```python
from build123d import *

# Parameters (mm, degrees)
SKETCH1_R           = 102.9
BOSS_EXTRUDE1_DEPTH = 230
BOSS_EXTRUDE1_DRAFT = -3
SHELL2_T            = -1


with BuildPart() as part:
    # Sketch1 → Boss-Extrude1 (with draft: the straight prism first)
    with BuildSketch(Plane(origin=(0, 0, 0), x_dir=(1, 0, 0), z_dir=(0, 1, 0))):
        Circle(SKETCH1_R)
    extrude(amount=BOSS_EXTRUDE1_DEPTH)
    # Boss-Extrude1: the draft: its side faces are tilted about the plane it starts from
    boss_extrude1_sides = [part.faces().sort_by_distance(p)[0] for p in [
        (-102.9, 115, 0),
    ]]
    draft(boss_extrude1_sides, Plane(origin=(0, 0, 0), x_dir=(1, 0, 0), z_dir=(0, 1, 0)), BOSS_EXTRUDE1_DRAFT)

    # Shell2
    shell2_openings = [part.faces().sort_by_distance(p)[0] for p in [
        (0, 230, 0),
    ]]
    offset(amount=SHELL2_T, openings=shell2_openings, kind=Kind.INTERSECTION)

    # Sketch4 → Revolve2 (revolve)
    with BuildSketch(Plane.XY, mode=Mode.PRIVATE) as revolve2_sk:
        Polygon((114.953789235, 230), (125.477867028, 230), (124.953789235, 220), (122.849117323, 220), (123.268523203, 228.00274093), (114.849117323, 228.00274093), align=None)
    revolve(revolve2_sk.sketch.rotate(Axis((0, 230, 0), (0, -1, 0)), 90), axis=Axis((0, 230, 0), (0, -1, 0)))


solid = part.part
```
CAD build for the part. Positions are in the model's coordinates, mm. A direction names the side the tool comes from. Round coordinates to 2 decimals unless told otherwise and drop trailing zeros. Write each loop counter-clockwise with the first axis right and the second up, starting at its lowest first coordinate (ties: lowest second). Pieces come first, ordered by that corner, then holes. Notation, with made-up numbers: (-23.75, 61) - (-4.75, 61) arc R20 cw to (-4.75, 81) - close; hole circle Ø1 at (-40, 47.5). An arc over 180 degrees is marked (long way). Write item = value, one per line. Start each with the question number.
Q1. Which spindle directions (+Z, -Z, +X, -X, +Y, -Y) get a long thin tool onto all of the face, cutting with end or side? Do faces 4 (the flat face through (83, 220, 92)), 5 (the flat face through (-1, 1, -1)), 6 (the conical face through (109.01, 220.5, 56.7)). Say none if no direction does.
Q2. Band-saw the part on B-B (x = 0). Give the cut face in (y, z).
Q3. Band-saw the part on C-C (z = 0). Give the cut face in (x, y), then the cut area to 3 significant figures.
Q4. Mould opens along Z. For faces 1 (the flat face through (-101, 228.003, -55)), 2 (the conical face through (122.01, 220.49, -27.09)), 3 (the flat face through (111, 230, -27)) say: pulls with the +Z half, pulls with the -Z half, needs draft (parallel to the pull), parting line crosses it, or undercut.
Q5. Band-saw the part on A-A (y = 122). Give the cut face in (x, z).
Q6. Drop flat-ended pins along their axis: pin 1 (6 mm diameter, centred on y = 128, z = 37, fed in from -X); pin 2 (5 mm diameter, centred on x = 55.5, y = 99.5, fed in from -Z); pin 3 (6 mm diameter, centred on y = 173.5, z = 15.5, fed in from +X). Give the stop position or say it passes through.
Q7. Probe L1, parallel to Y at x = -22, z = -64; L2, parallel to Z at x = -29, y = 144; L3, parallel to Z at x = 8.5, y = 209.5. List the from-to ranges inside material, lowest first. Write a range as from..to.
Q8. Band-saw the part on D-D (y = 69). Give the cut face in (x, z), then the cut area to 3 significant figures.
Answers below:
q1.face_4 = -Y
q1.face_5 = +Y
q1.face_6 = none
q2.outline = (0, -102.9) - (228, -114.85) - (228, -123.27) - (220, -122.85) - (220, -124.95) - (230, -125.48) - (230, -113.95) - (1, -101.95) - (1, 101.95) - (230, 113.95) - (230, 125.48) - (220, 124.95) - (220, 122.85) - (228, 123.27) - (228, 114.85) - (0, 102.9) - close
q3.outline = (-125.48, 230) - (-124.95, 220) - (-122.85, 220) - (-123.27, 228) - (-114.85, 228) - (-102.9, 0) - (102.9, 0) - (114.85, 228) - (123.27, 228) - (122.85, 220) - (124.95, 220) - (125.48, 230) - (113.95, 230) - (101.95, 1) - (-101.95, 1) - (-113.95, 230) - close
q3.area = 740 mm2
q4.face_1 = undercut
q4.face_2 = parting line crosses it
q4.face_3 = needs draft
q5.outline = circle Ø218.59 at (0, 0); hole circle Ø216.58 at (0, 0)
q6.pin_1 = -104.22
q6.pin_2 = -94.24
q6.pin_3 = 111.33
q7.L1 = 0..1
q7.L2 = -106.57..-105.53, 105.53..106.57
q7.L3 = -113.56..-112.56, 112.56..113.56
q8.outline = circle Ø213.03 at (0, 0); hole circle Ø211.03 at (0, 0)
q8.area = 667 mm2
